Can you work these out from the model? Positions are in its coordinate system, mm. A direction names the side the tool comes from. Give positions to 0.01 mm unless a question says otherwise; leave off trailing zeros. Write each loop counter-clockwise with the first axis right and the second up, starting at its lowest first coordinate (ties: lowest second). Pieces come first, ordered by that corner, then holes.
1. Suppose I cut it at C-C (x = -3.5). Please give me the cut outline in (y, z) (3 decimals), and give its area (3 significant figures).
2. Suppose I cut it at B-B (z = 0.75). Please give me the cut outline in (x, y) (3 decimals).
3. Suppose I cut it at D-D (y = 2.75). Please give me the cut outline in (x, z) (3 decimals).
4. If I drill on probe 1 along X at (y, z) = (4.25, -4.5) (3 decimals); probe 2 along Z at (x, y) = (-29.5, 0.25); probe 3 along Z at (x, y) = (-26, -0.25), over which ranges is the centre line in solid material (lowest first)?
5. On a 3-axis mill with a long thin cutter (end or side, diameter ignored), from which of +Z, -Z, +X, -X, +Y, -Y can I reach the whole of each face in a straight line? I mean faces 1 (the cylindrical face through (6, -2, 0)), 2 (the cylindrical face through (-30.14, -6.2, -1.38)). Say none if no direction works.
6. Suppose I cut it at A-A (y = 0). Please give me the cut outline in (x, z) (3 decimals), and give its area (3 significant figures).
7. I'm going to push flat-ended pins straight in: pin 1 (2 mm diameter, centred on x = -8, y = -3.5, fed in from -Z); pin 2 (1.5 mm diameter, centred on x = -6, y = -3.5, fed in from -Z); pin 3 (6 mm diameter, centred on x = -5.5, y = -2, fed in from -Z) (3 decimals); pin 4 (1.5 mm diameter, centred on x = 1.5, y = 3.5, fed in from -Z). Where does each tip first touch, or does it pass through?
```python
from build123d import *

# Parameters (mm, degrees)
SKETCH1_R           = 2
BOSS_EXTRUDE1_DEPTH = 11.43
BOSS_EXTRUDE2_START = -28.575
SKETCH1_3_R         = 3.175
SKETCH1_3_R_2       = 2
BOSS_EXTRUDE2_DEPTH = 28.575
SKETCH2_R           = 6.35
BOSS_EXTRUDE3_DEPTH = 3.175


with BuildPart() as part:
    # Sketch1 → Boss-Extrude1 (new body)
    with BuildSketch(Plane(origin=(0, 0, 0), x_dir=(0, 0, -1), z_dir=(1, 0, 0))):
        Circle(SKETCH1_R)
    extrude(amount=BOSS_EXTRUDE1_DEPTH)

    # Sketch1_3 → Boss-Extrude2 (add)
    with BuildSketch(Plane(origin=(0, 0, 0), x_dir=(0, 0, -1), z_dir=(1, 0, 0)).offset(BOSS_EXTRUDE2_START)):
        Circle(SKETCH1_3_R)
        Circle(SKETCH1_3_R_2)
    extrude(amount=BOSS_EXTRUDE2_DEPTH)

    # Sketch2 → Boss-Extrude3 (add)
    with BuildSketch(Plane.ZY.offset(28.575)):
        Circle(SKETCH2_R)
    extrude(amount=BOSS_EXTRUDE3_DEPTH)


solid = part.part
```
Checks:
1. outline: circle Ø6.35 at (0, 0)
1. area: 31.7 mm2
2. outline: (-31.75, -6.306) - (-28.575, -6.306) - (-28.575, -3.085) - (0, -3.085) - (0, -1.854) - (11.43, -1.854) - (11.43, 1.854) - (0, 1.854) - (0, 3.085) - (-28.575, 3.085) - (-28.575, 6.306) - (-31.75, 6.306) - close
3. outline: (-31.75, -5.724) - (-28.575, -5.724) - (-28.575, -1.587) - (0, -1.587) - (0, 1.587) - (-28.575, 1.587) - (-28.575, 5.724) - (-31.75, 5.724) - close
4. probe 1: x = -31.75 to -28.575
4. probe 2: z = -6.35 to 6.35
4. probe 3: z = -3.17 to 3.17
5. face 1: +X
5. face 2: +X, -X
6. outline: (-31.75, -6.35) - (-28.575, -6.35) - (-28.575, -3.175) - (0, -3.175) - (0, -2) - (11.43, -2) - (11.43, 2) - (0, 2) - (0, 3.175) - (-28.575, 3.175) - (-28.575, 6.35) - (-31.75, 6.35) - close
6. area: 267 mm2
7. pin 1: stops at z = -1.96
7. pin 2: stops at z = -1.59
7. pin 3: stops at z = -3.175
7. pin 4: passes through
